Autodesk Inventor part; units mm, degrees
ref_plane "YZ Plane" through (0, 0, 0) normal (1, 0, 0) x (0, 1, 0)
ref_plane "XZ Plane" through (0, 0, 0) normal (0, 1, 0) x (-1, 0, 0)
ref_plane "XY Plane" through (0, 0, 0) normal (0, 0, 1) x (1, 0, 0)
sketch "Sketch1" plane through (0, 0, 0) normal (0, 0, 1) x (1, 0, 0)
  line L0 (0, 0) -> (16, 0)
  line L1 (16, 0) -> (16, 8)
  line L2 (16, 8) -> (0, 8)
  line L3 (0, 8) -> (0, 0)
  dimension "d0" = 16
  dimension "d1" = 8
extrude "Extrusion1" add sketch "Sketch1" against normal blind 9.6
sketch "Sketch2" plane through (0, 0, 0) normal (0, 0, 1) x (1, 0, 0)
  circle A0 centre (3.8, 4.2) radius 2.4
  circle A1 centre (11.8, 4.2) radius 2.4
  line L0 (16, 8) -> (0, 8)
  line L1 (0, 0) -> (0, 8)
  dimension "d4" = 4.8
  dimension "d5" = 4.8
  dimension "d6" = 3.8
  dimension "d7" = 3.8
  dimension "d8" = 8
extrude "Extrusion2" add sketch "Sketch2" along normal blind 1.8
sketch "Sketch3" plane through (0, 0, -9.6) normal (0, 0, -1) x (-1, 0, 0)
  line L0 (-14.8, 6.8) -> (-1.2, 6.8)
  line L1 (-1.2, 6.8) -> (-1.2, 1.2)
  line L2 (-1.2, 1.2) -> (-14.8, 1.2)
  line L3 (-14.8, 1.2) -> (-14.8, 6.8)
  line L4 (-16, 8) -> (0, 8)
  line L5 (-16, 0) -> (-16, 8)
  line L6 (-16, 0) -> (0, 0)
  line L7 (0, 0) -> (0, 8)
  circle A0 centre (-8, 4) radius 1
  dimension "d11" = 1.2
  dimension "d12" = 1.2
  dimension "d13" = 1.2
  dimension "d14" = 1.2
  dimension "d15" = 2
  dimension "d16" = 8
  dimension "d17" = 4
extrude "Extrusion3" cut sketch "Sketch3" against normal blind 1.8 contours L0 L1 L2 L3
sketch "Sketch4" plane through (0, 8, 0) normal (0, 1, 0) x (1, 0, 0)
  line L0 (0, 9.6) -> (16, 9.6)
  line L1 (14.8, 7.8) -> (1.2, 7.8)
  line L2 (0, 0) -> (0, 9.6)
  point P0 (8, 5)
  dimension "d21" = 2.8
  dimension "d22" = 8
hole "Hole1" at (8, 8, -5) direction (0, -1, 0) diameter 4.8 depth 25.4 tip angle 118
properties part number "Yee_1x2BrickWithHole"
Check sheet for the modelled part. Datum: model origin and axes. Units: mm. A direction names the side the tool comes from. Give positions to 0.01 mm unless a question says otherwise; leave off trailing zeros. Order: outer loops, then holes, each group sorted by start corner. A loop starts at its lowest first (then second) coordinate and runs counter-clockwise, first axis right, second up. Notation, with made-up numbers: M 31.5,26 L 52.5,26 A18 ccw 52.5,59 Z; hole C 86.5,-33 d8. An arc over 180 degrees is marked long. Answer in a Markdown table with one row per item. Add a question column.
Q1. Gauge pin test, flat ends, axial feed: pin 1 Ø1.5 at (x, y) = (7, 2) entering from +Z; pin 2 Ø1.5 at (x, y) = (5.5, 4.5) entering from -Z. Record the tip position at first contact, or that the pin passes through.
Q2. Thickness scan on L1, parallel to X at y = 6.5, z = -5; L2, parallel to X at y = 2.75, z = -8.25; L3, parallel to Y at x = 14.25, z = -8.75. Record the ranges inside material, lowest first.
Q3. Sectioned sample at C-C, the plane y = 1.5. Record the boundary of the cut face in (x, z), and give its area (3 significant figures).
Q4. Release check for a two-part mould opening along Y. For faces 4 (the flat face through (10, 8, -3)), 5 (the flat face through (8, 6.8, -9)), 6 (the flat face through (8, 1, -9.6)) record: released by +Y, released by -Y, zero draft, split by the parting line, or undercut.
Q5. Sectioned sample at A-A, the plane z = -5. Record the boundary of the cut face in (x, y), and give its area (3 significant figures).
Q6. Access from +Z, -Z, +X, -X, +Y, -Y to the whole of each face (thin tool, end or side, straight path). Record for faces 1 (the cylindrical face through (14.09, 3.48, 0.89)), 2 (the flat face through (4, 4, 1.8)), 3 (the flat face through (1.2, 4, -9)).
Q7. Sectioned sample at D-D, the plane x = 3.8. Record the boundary of the cut face in (y, z).
Q8. Sectioned sample at B-B, the plane x = 8. Record the boundary of the cut face in (y, z).
Verdict:
| question | item | result |
|---|---|---|
| 1 | pin 1 | z = 0 |
| 1 | pin 2 | z = -7.8 |
| 2 | L1 | 0 to 5.6, 10.4 to 16 |
| 2 | L2 | 0 to 1.2, 14.8 to 16 |
| 2 | L3 | 0 to 1.2, 6.8 to 8 |
| 3 | outline | M 0,-9.6 L 1.2,-9.6 L 1.2,-7.8 L 14.8,-7.8 L 14.8,-9.6 L 16,-9.6 L 16,0 L 0,0 Z; hole C 8,-5 d4.8 |
| 3 | area | 111 mm² |
| 4 | face 4 | released by +Y |
| 4 | face 5 | undercut |
| 4 | face 6 | zero draft |
| 5 | outline | M 0,0 L 5.6,0 L 5.6,8 L 0,8 Z; M 10.4,0 L 16,0 L 16,8 L 10.4,8 Z |
| 5 | area | 89.6 mm² |
| 6 | face 1 | +Z |
| 6 | face 2 | +Z, +X, -X, +Y, -Y |
| 6 | face 3 | -Z |
| 7 | outline | M 0,-9.6 L 1.2,-9.6 L 1.2,-7.8 L 6.8,-7.8 L 6.8,-9.6 L 8,-9.6 L 8,0 L 6.6,0 L 6.6,1.8 L 1.8,1.8 L 1.8,0 L 0,0 Z |
| 8 | outline | M 0,-9.6 L 1.2,-9.6 L 1.2,-7.8 L 3,-7.8 L 3,-9.6 L 5,-9.6 L 5,-7.8 L 6.8,-7.8 L 6.8,-9.6 L 8,-9.6 L 8,-7.4 L 0,-7.4 Z; M 0,-2.6 L 8,-2.6 L 8,0 L 0,0 Z |
